Geometry check sheet. Reference: the model listing, model coordinates, mm. Face numbers are marked on the shaded views. A direction names the side the tool comes from. Round coordinates to 2 decimals unless told otherwise and drop trailing zeros. Write each loop counter-clockwise with the first axis right and the second up, starting at its lowest first coordinate (ties: lowest second). Pieces come first, ordered by that corner, then holes. Notation, with made-up numbers: (27, 33) -> (34, 33) arc R21 ccw to (34, 41) -> close; hole circle Ø5 at (-30, -35). An arc over 180 degrees is marked (long way). Return JSON: item names as keys, results as strings. Group by question number.
from build123d import *

# Parameters (mm, degrees)
BOSS_EXTRUDE1_DEPTH            = 10
CUT_EXTRUDE1_REACH             = 52.408
SKETCH2_R                      = 8.25
M2_CLEARANCE_HOLE1_D           = 2.4
CBORE_FOR_M3_SHCS1_D           = 3.4
CBORE_FOR_M3_SHCS1_CBORE_D     = 6.5
CBORE_FOR_M3_SHCS1_CBORE_DEPTH = 3
CUT_EXTRUDE2_REACH             = 52.408
SKETCH7_W                      = 4
SKETCH7_H                      = 11
FILLET1_R                      = 1


with BuildPart() as part:
    # Sketch1 → Boss-Extrude1 (new, symmetric)
    with BuildSketch(Plane(origin=(0, 0, 0), x_dir=(0, 0, -1), z_dir=(1, 0, 0))):
        Polygon((29, 40), (26, 40), (26, 6), (3, 6), (3, 40), (0, 40), (0, 0), (29, 0), align=None)
    extrude(amount=BOSS_EXTRUDE1_DEPTH, both=True)

    # Sketch2 → Cut-Extrude1 (cut, up to next)
    with BuildSketch(Plane.XY, mode=Mode.PRIVATE) as cut_extrude1_sk1:
        with Locations((0, 30.5)):
            Circle(SKETCH2_R)
    cut_extrude1_tool1 = extrude(cut_extrude1_sk1.sketch, amount=-CUT_EXTRUDE1_REACH, mode=Mode.PRIVATE) & part.part
    add(cut_extrude1_tool1.solids().sort_by_distance((0, 30.5, 0))[0], mode=Mode.SUBTRACT)

    # M2 Clearance Hole1 (through all)
    with Locations(Plane.XY):
        with Locations((-8, 8), (8, 8), (8, 38), (-8, 38)):
            Hole(M2_CLEARANCE_HOLE1_D / 2)

    # CBORE for M3 SHCS1 (through all)
    with Locations(Plane(origin=(0, 6, 0), x_dir=(1, 0, 0), z_dir=(0, 1, 0))):
        with Locations((0, 19.5), (0, 9.5)):
            CounterBoreHole(CBORE_FOR_M3_SHCS1_D / 2, CBORE_FOR_M3_SHCS1_CBORE_D / 2, CBORE_FOR_M3_SHCS1_CBORE_DEPTH)

    # Sketch7 → Cut-Extrude2 (cut, up to next)
    with BuildSketch(Plane.XY.offset(-29), mode=Mode.PRIVATE) as cut_extrude2_sk1:
        with Locations((8, 21.5)):
            Rectangle(SKETCH7_W, SKETCH7_H)
    cut_extrude2_tool1 = extrude(cut_extrude2_sk1.sketch, amount=CUT_EXTRUDE2_REACH, mode=Mode.PRIVATE) & part.part
    # Sketch7 → Cut-Extrude2 (cut, up to next)
    with BuildSketch(Plane.XY.offset(-29), mode=Mode.PRIVATE) as cut_extrude2_sk2:
        with Locations((-8, 21.5)):
            Rectangle(SKETCH7_W, SKETCH7_H)
    cut_extrude2_tool2 = extrude(cut_extrude2_sk2.sketch, amount=CUT_EXTRUDE2_REACH, mode=Mode.PRIVATE) & part.part
    add(cut_extrude2_tool1.solids().sort_by_distance((8, 21.5, -29))[0], mode=Mode.SUBTRACT)
    add(cut_extrude2_tool2.solids().sort_by_distance((-8, 21.5, -29))[0], mode=Mode.SUBTRACT)

    # Fillet1
    fillet1_edges = [part.edges().sort_by_distance(p)[0] for p in [
        (-6, 27, -27.5),
        (-10, 27, -27.5),
        (-10, 16, -27.5),
        (-6, 16, -27.5),
        (-10, 40, -1.5),
        (-10, 40, -27.5),
        (0, 0, -29),
        (0, 0, 0),
        (10, 40, -1.5),
        (10, 40, -27.5),
        (10, 16, -27.5),
        (10, 27, -27.5),
        (6, 27, -27.5),
        (6, 16, -27.5),
    ]]
    fillet(fillet1_edges, radius=FILLET1_R)


solid = part.part
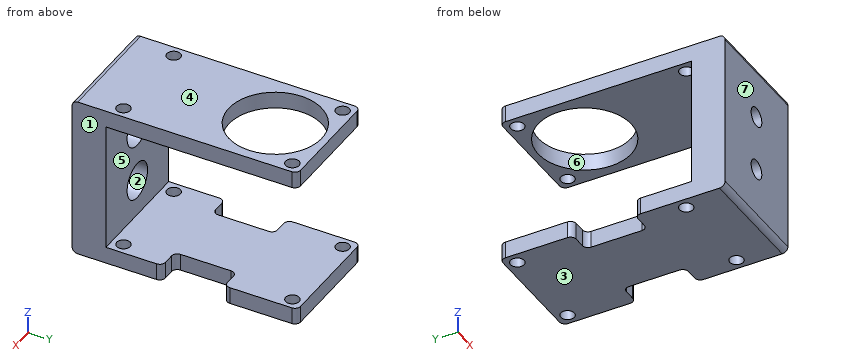
1) Mould release check, pull along Z, two halves, no side actions. Record for the marked faces 1, 2, 3 and 4: +Z half, -Z half, draft (parallel to the pull), parting line (faces both ways), or undercut.
2) Go/stop test with flat-tipped pins: P1, Ø2.5, axis at x = 0, z = -9.5, coming from the +Y side; P2, Ø2, axis at x = -1, z = -19, coming from the +Y side; P3, Ø1, axis at x = 7, z = -12, coming from the +Y side. Record where each tip stops, or that it passes through.
3) Material ranges on probe 1 along Z at (x, y) = (-5.25, 37); probe 2 along Y at (x, z) = (-7.75, -19); probe 3 along Y at (x, z) = (0, -1.7), recorded low to high. Write a range as [from, to].
4) Sectioned sample at D-D on y = 12. Enter the section's corners in (x, z), and give its area (3 significant figures).
5) Sectioned sample at B-B on z = -2. Enter the section's corners in (x, y), and give its area (3 significant figures).
6) Tool access check on the marked faces 5, 6 and 7. Record the directions out of +Z, -Z, +X, -X, +Y, -Y that give a thin tool (end or side, any length) a straight path to the whole face; none if there is none.
7) Sectioned sample at A-A on y = 8. Enter the section's corners in (x, z).
8) Sectioned sample at C-C on z = -9.5. Enter the section's corners in (x, y).
Evaluation:
{
 "1": {"face 1": "draft", "face 2": "undercut", "face 3": "-Z half", "face 4": "+Z half"},
 "2": {"P1": "passes through", "P2": "stops at y = 3", "P3": "stops at y = 6"},
 "3": {"probe 1": "z = [-29, -26], [-3, 0]", "probe 2": "y = [0, 6]", "probe 3": "y = [0, 22.25], [38.75, 40]"},
 "4": {"outline": "(-10, -29) -> (10, -29) -> (10, -26) -> (-10, -26) -> close; (-10, -3) -> (10, -3) -> (10, 0) -> (-10, 0) -> close", "area": "120 mm2"},
 "5": {"outline": "(-10, 0) -> (10, 0) -> (10, 39) arc R1 ccw to (9, 40) -> (-9, 40) arc R1 ccw to (-10, 39) -> close; hole circle Ø2.4 at (-8, 8); hole circle Ø2.4 at (-8, 38); hole circle Ø16.5 at (0, 30.5); hole circle Ø2.4 at (8, 8); hole circle Ø2.4 at (8, 38)", "area": "568 mm2"},
 "6": {"face 5": "+X, -X, +Y", "face 6": "+Z", "face 7": "+Z, -Z, +X, -X, -Y"},
 "7": {"outline": "(-10, -29) -> (-9.2, -29) -> (-9.2, -26) -> (-10, -26) -> close; (-10, -3) -> (-9.2, -3) -> (-9.2, 0) -> (-10, 0) -> close; (-6.8, -29) -> (6.8, -29) -> (6.8, -26) -> (-6.8, -26) -> close; (-6.8, -3) -> (6.8, -3) -> (6.8, 0) -> (-6.8, 0) -> close; (9.2, -29) -> (10, -29) -> (10, -26) -> (9.2, -26) -> close; (9.2, -3) -> (10, -3) -> (10, 0) -> (9.2, 0) -> close"},
 "8": {"outline": "(-10, 0) -> (-1.7, 0) -> (-1.7, 3) -> (-3.25, 3) -> (-3.25, 6) -> (-10, 6) -> close; (1.7, 0) -> (10, 0) -> (10, 6) -> (3.25, 6) -> (3.25, 3) -> (1.7, 3) -> close"}
}
